Part model, mm, in its own coordinate system. A direction names the side the tool comes from. Round coordinates to 2 decimals unless told otherwise and drop trailing zeros. Order: outer loops, then holes, each group sorted by start corner. A loop starts at its lowest first (then second) coordinate and runs counter-clockwise, first axis right, second up. Notation, with made-up numbers: (5, -33) -> (34, -33) arc R26 ccw to (34, -5) -> close; hole circle Ø6 at (57.25, -15). An arc over 180 degrees is marked (long way). Answer as a JSON object with one key per item and string values. Group by question number.
```python
from build123d import *

# Parameters (mm, degrees)
CYLINDER008_R     = 2
CYLINDER008_DEPTH = 4
CYLINDER015_R     = 2
CYLINDER015_DEPTH = 4
BOX006_W          = 34
BOX006_H          = 23
BOX006_DEPTH      = 2
BOX003_W          = 52
BOX003_H          = 25.6
BOX003_DEPTH      = 2


with BuildPart() as button_hole:
    # Cylinder008 → Cylinder008 (new body)
    with BuildSketch(Plane(origin=(50, 7, 38), x_dir=(1, 0, 0), z_dir=(0, 0, 1))):
        Circle(CYLINDER008_R)
    extrude(amount=CYLINDER008_DEPTH)


with BuildPart() as button_hole001:
    # Cylinder015 → Cylinder015 (new body)
    with BuildSketch(Plane(origin=(50, 22, 38), x_dir=(1, 0, 0), z_dir=(0, 0, 1))):
        Circle(CYLINDER015_R)
    extrude(amount=CYLINDER015_DEPTH)


with BuildPart() as fusion004:
    # Box006 → Box006 (new body)
    with BuildSketch(Plane(origin=(5, 5, 40), x_dir=(1, 0, 0), z_dir=(0, 0, 1))):
        with Locations((17, 11.5)):
            Rectangle(BOX006_W, BOX006_H)
    extrude(amount=BOX006_DEPTH)

    # Fusion004: union button_hole, button_hole001
    add(button_hole.part)
    add(button_hole001.part)


with BuildPart() as cover:
    # Box003 → Box003 (new body)
    with BuildSketch(Plane(origin=(2, 2, 40), x_dir=(1, 0, 0), z_dir=(0, 0, 1))):
        with Locations((26, 12.8)):
            Rectangle(BOX003_W, BOX003_H)
    extrude(amount=BOX003_DEPTH)

    # Cut: cut Fusion004
    add(fusion004.part, mode=Mode.SUBTRACT)


solid = cover.part
```
Q1. Band-saw the part on C-C (y = 12). List the corners of the cut face in (x, z).
Q2. Band-saw the part on A-A (x = 50). List the corners of the cut face in (y, z), plus the area to 3 significant figures.
Q3. Drop flat-ended pins along their axis: pin 1 Ø0.6 at (x, z) = (26, 41) entering from +Y; pin 2 Ø3 at (x, y) = (50, 7) entering from +Z. Give the stop position or say it passes through.
Q4. Wall check: line 1 (Y direction, x = 50, z = 40.6); line 2 (X direction, y = 7, z = 40.8); line 3 (X direction, y = 19.5, z = 41.65). Give the ranges that are in metal, low to high. Write a range as [from, to].
Q5. Which spindle directions (+Z, -Z, +X, -X, +Y, -Y) get a long thin tool onto all of the face, cutting with end or side? Do faces 4 (the flat face through (39, 16, 41)), 5 (the flat face through (3, 27.6, 41)). Say none if no direction does.
Q6. Band-saw the part on D-D (z = 41.25). List the corners of the cut face in (x, y), plus the area to 3 significant figures.
Q7. Band-saw the part on B-B (y = 22). List the corners of the cut face in (x, z), plus the area to 3 significant figures.
Q8. Two-plate mould, pull along X, no slides. Class faces 1 (the flat face through (46, 27.6, 41)), 2 (the flat face through (22, 5, 41)), 3 (the flat face through (2, 15, 41)): +X half, -X half, draft (parallel to the pull), parting line (faces both ways), or undercut.
Completed:
{
 "1": {"outline": "(2, 40) -> (5, 40) -> (5, 42) -> (2, 42) -> close; (39, 40) -> (54, 40) -> (54, 42) -> (39, 42) -> close"},
 "2": {"outline": "(2, 40) -> (5, 40) -> (5, 42) -> (2, 42) -> close; (9, 40) -> (20, 40) -> (20, 42) -> (9, 42) -> close; (24, 40) -> (27.6, 40) -> (27.6, 42) -> (24, 42) -> close", "area": "35.2 mm2"},
 "3": {"pin 1": "y = 5", "pin 2": "through"},
 "4": {"line 1": "[2, 5], [9, 20], [24, 27.6]", "line 2": "[2, 5], [39, 48], [52, 54]", "line 3": "[2, 5], [39, 54]"},
 "5": {"face 4": "+Z, -Z, +Y", "face 5": "+Z, -Z, +X, -X, +Y"},
 "6": {"outline": "(2, 2) -> (54, 2) -> (54, 27.6) -> (39, 27.6) -> (39, 5) -> (5, 5) -> (5, 27.6) -> (2, 27.6) -> close; hole circle Ø4 at (50, 7); hole circle Ø4 at (50, 22)", "area": "538 mm2"},
 "7": {"outline": "(2, 40) -> (5, 40) -> (5, 42) -> (2, 42) -> close; (39, 40) -> (48, 40) -> (48, 42) -> (39, 42) -> close; (52, 40) -> (54, 40) -> (54, 42) -> (52, 42) -> close", "area": "28.0 mm2"},
 "8": {"face 1": "draft", "face 2": "undercut", "face 3": "-X half"}
}
